Build history of the part. All positions in model axes, mm. A direction names the side the tool comes from. Round coordinates to 2 decimals unless told otherwise and drop trailing zeros. Write each loop counter-clockwise with the first axis right and the second up, starting at its lowest first coordinate (ties: lowest second). Pieces come first, ordered by that corner, then holes.
1) Wall check: probe 1 along Z at (x, y) = (37, 11.75); probe 2 along X at (y, z) = (11.25, -39); probe 3 along Y at (x, z) = (25, 4). Give the ranges that are in metal, low to high.
2) Pull direction Z, two halves, no side cores. Call faces 4 (the flat face through (-64, 12, 1)), 5 (the flat face through (-1, 12, -43)), 6 (the flat face through (-1, 0, -1)), 7 (the flat face through (65.812, 18.042, 2.155)): +Z half, -Z half, draft (parallel to the pull), parting line (faces both ways), or undercut.
3) Flat gauge pins, fed straight in: pin 1 (1.3 mm diameter, centred on y = 17, z = -0.5, fed in from +X); pin 2 (2.5 mm diameter, centred on y = 19.5, z = -0.5, fed in from +X); pin 3 (6 mm diameter, centred on x = 22.5, z = 31.5, fed in from +Y). Where does each tip first touch, or does it go through?
4) Saw through at B-B (x = 21). Write the cut outline in (y, z).
5) Saw through at A-A (z = -18). Write the cut outline in (x, y).
6) Which spindle directions (+Z, -Z, +X, -X, +Y, -Y) get a long thin tool onto all of the face, cutting with end or side? Do faces 1 (the flat face through (-64.5, 18, 0)), 2 (the flat face through (-1, 8, -1)), 3 (the flat face through (-1, 7, -47.5)). Say none if no direction does.
from build123d import *

# Parameters (mm, degrees)
SKETCH1_W           = 138
SKETCH1_H           = 95
BOSS_EXTRUDE1_DEPTH = 15
SKETCH2_W           = 128
SKETCH2_H           = 86
CUT_EXTRUDE1_DEPTH  = 7
SNAP_START          = 64.5
SNAP_HOOK2_DEPTH    = 2
SNAP_HOOK2_2_DEPTH  = 2
FILLET1_R           = 1
FILLET2_R           = 0.5


with BuildPart() as part:
    # Sketch1 → Boss-Extrude1 (new body)
    with BuildSketch(Plane(origin=(0, 0, 0), x_dir=(1, 0, 0), z_dir=(0, 1, 0))):
        Rectangle(SKETCH1_W, SKETCH1_H)
    extrude(amount=BOSS_EXTRUDE1_DEPTH)

    # Sketch2 → Cut-Extrude1 (cut)
    with BuildSketch(Plane(origin=(0, 15, 0), x_dir=(1, 0, 0), z_dir=(0, 1, 0))):
        Rectangle(SKETCH2_W, SKETCH2_H)
    extrude(amount=-CUT_EXTRUDE1_DEPTH, mode=Mode.SUBTRACT)



with BuildPart() as body_2:
    # Snap Hook2: read off the stored shape, not the designer's step
    # Snap Hook2 outline → Snap Hook2 (new body)
    with BuildSketch(Plane.YZ.offset(SNAP_START)):
        Polygon((21, -2), (21, 2), (18, 2.157223338), (18, -2.157223338), align=None)
    snap_hook2 = extrude(amount=SNAP_HOOK2_DEPTH)


with BuildPart() as part_1:
    add(part.part)

    add(body_2.part)  # Snap Hook2 2 merges body 2
    # Snap Hook2 2 outline → Snap Hook2 2 (add)
    with BuildSketch(Plane.YZ.offset(SNAP_START)):
        Polygon((18, -2.157223338), (18, 2.157223338), (15, 2.314446676), (15, -2.314446676), align=None)
    snap_hook2_2 = extrude(amount=SNAP_HOOK2_2_DEPTH)

    # Snap Hook2 3: loft between two sections, ruled curve by curve
    snap_hook2_3_from = [
        Edge.make_line((66.5, 21, -2), (66.5, 21, 2)),
        Edge.make_line((66.5, 18, 2.157223338), (66.5, 18, -2.157223338)),
        Edge.make_line((66.5, 18, 2.157223338), (66.5, 21, 2)),
        Edge.make_line((66.5, 18, -2.157223338), (66.5, 21, -2)),
    ]
    snap_hook2_3_to = [
        Edge.make_line((68.5, 19, -2.104815559), (68.5, 19, 2.104815559)),
        Edge.make_line((68.5, 18, 2.157223338), (68.5, 18, -2.157223338)),
        Edge.make_line((68.5, 18, 2.157223338), (68.5, 19, 2.104815559)),
        Edge.make_line((68.5, 18, -2.157223338), (68.5, 19, -2.104815559)),
    ]
    snap_hook2_3 = Solid(Shell([*[Face.make_surface_from_curves(snap_hook2_3_from[k], snap_hook2_3_to[k]) for k in range(4)], Face(Wire(snap_hook2_3_from)), Face(Wire(snap_hook2_3_to))]))
    add(snap_hook2_3)

    # Fillet1
    fillet1_edges = [part_1.edges().sort_by_distance(p)[0] for p in [
        (64, 11.5, -43),
        (64, 11.5, 43),
        (-64, 11.5, 43),
        (-64, 11.5, -43),
        (-69, 7.5, -47.5),
        (69, 7.5, -47.5),
        (69, 7.5, 47.5),
        (-69, 7.5, 47.5),
    ]]
    fillet(fillet1_edges, radius=FILLET1_R)

    # Mirror1: Snap Hook2, Snap Hook2 2, Snap Hook2 3 across plane
    add(snap_hook2.mirror(Plane(origin=(0, 0, 0), x_dir=(0, 0, 1), z_dir=(1, 0, 0))))
    add(snap_hook2_2.mirror(Plane(origin=(0, 0, 0), x_dir=(0, 0, 1), z_dir=(1, 0, 0))))
    add(snap_hook2_3.mirror(Plane(origin=(0, 0, 0), x_dir=(0, 0, 1), z_dir=(1, 0, 0))))

    # Fillet2
    fillet2_edges = [part_1.edges().sort_by_distance(p)[0] for p in [
        (66.5, 15, 0),
        (64.5, 15, 0),
        (-66.5, 15, 0),
        (-64.5, 15, 0),
    ]]
    fillet(fillet2_edges, radius=FILLET2_R - 0.0001)  # a hair under: the kernel refuses the full size


solid = part_1.part
Evaluation:
1. probe 1: z = -47.5 to -43, 43 to 47.5
1. probe 2: x = -69 to -64, 64 to 69
1. probe 3: y = 0 to 8
2. face 4: undercut
2. face 5: undercut
2. face 6: draft
2. face 7: +Z half
3. pin 1: stops at x = 66.5
3. pin 2: stops at x = 68.5
3. pin 3: stops at y = 8
4. outline: (0, -47.5) - (15, -47.5) - (15, -43) - (8, -43) - (8, 43) - (15, 43) - (15, 47.5) - (0, 47.5) - close
5. outline: (-69, 0) - (69, 0) - (69, 15) - (64, 15) - (64, 8) - (-64, 8) - (-64, 15) - (-69, 15) - close
6. face 1: +Z, -Z, +Y
6. face 2: +Y
6. face 3: -Z, +X, -X, +Y, -Y
